Read the model definition and answer for the solid it produces. Units are mm, in the model's axes. Face numbers are marked on the shaded views. A direction names the side the tool comes from. Coordinates: 2 decimals unless noted, no trailing zeros. Loops run counter-clockwise (first coordinate to the right, second up) from the corner with the lowest first, then second, coordinate; pieces in that order, holes last. Notation, with made-up numbers: M -19,-20 L -5,-20 A26 ccw -5,-6 Z; hole C -12.5,36 d10. An arc over 180 degrees is marked long. Put each result on its own line as item: value.
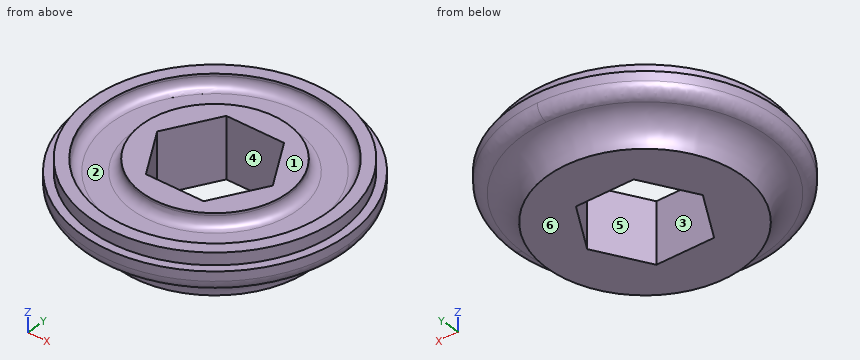
from build123d import *

# Parameters (mm, degrees)
SKETCH1_R                         = 17.4625
HEX_AXEL_CUTOUT_OUTSIDE_RIM_DEPTH = 15.875
SKETCH3_R                         = 19.05
SKETCH3_R_2                       = 16.383
PIPE_STEP_DEPTH                   = 1.5875
SKETCH5_R                         = 14.7955
SKETCH5_R_2                       = 9.525
SPOKE_STEP_DEPTH                  = 1.5875
FILLET1_R                         = 1.27
FILLET2_R                         = 1.5875
SKETCH7_W                         = 50.409195303
SKETCH7_H                         = 73.287011446
MIDCUT_DEPTH                      = 8.9375


with BuildPart() as part:
    # Sketch1 → Hex Axel Cutout & Outside Rim (new body)
    with BuildSketch(Plane.XY):
        Circle(SKETCH1_R)
        Polygon((-7.522989478, 0), (-3.761494739, -6.5151), (3.761494739, -6.5151), (7.522989478, 0), (3.761494739, 6.5151), (-3.761494739, 6.5151), align=None, mode=Mode.SUBTRACT)
    extrude(amount=HEX_AXEL_CUTOUT_OUTSIDE_RIM_DEPTH)

    # Sketch3 → Pipe Step (cut)
    with BuildSketch(Plane.XY.offset(15.875)):
        Circle(SKETCH3_R)
        Circle(SKETCH3_R_2, mode=Mode.SUBTRACT)
    pipe_step = extrude(amount=-PIPE_STEP_DEPTH, mode=Mode.SUBTRACT)

    # Step Mirror: Pipe Step across plane
    add(pipe_step.mirror(Plane.XY.offset(7.9375)), mode=Mode.SUBTRACT)

    # Sketch4 → Poly Cord Groove (revolve, cut)
    with BuildSketch(Plane(origin=(0, 0, 0), x_dir=(0, 0, -1), z_dir=(1, 0, 0))):
        with BuildLine():
            Line((-4.3815, 16.331738244), (-4.3815, 17.4625))
            Line((-4.3815, 17.4625), (-11.4935, 17.4625))
            Line((-11.4935, 17.4625), (-11.4935, 16.331738244))
            ThreePointArc((-11.4935, 16.331738244), (-7.9375, 12.775738244), (-4.3815, 16.331738244))
        make_face()
    revolve(axis=Axis((0, 0, 14.2875), (0, 0, -1)), mode=Mode.SUBTRACT)

    # Sketch5 → Spoke Step (cut)
    with BuildSketch(Plane(origin=(0, 0, 0), x_dir=(-1, 0, 0), z_dir=(0, 0, -1))):
        Circle(SKETCH5_R)
        Circle(SKETCH5_R_2, mode=Mode.SUBTRACT)
    spoke_step = extrude(amount=-SPOKE_STEP_DEPTH, mode=Mode.SUBTRACT)

    # Spoke Step Mirror: Spoke Step across plane
    add(spoke_step.mirror(Plane.XY.offset(7.9375)), mode=Mode.SUBTRACT)

    # Fillet1
    fillet1_edges = [part.edges().sort_by_distance(p)[0] for p in [
        (14.7955, 0, 1.5875),
        (9.525, 0, 1.5875),
        (14.7955, 0, 14.2875),
        (9.525, 0, 14.2875),
    ]]
    fillet(fillet1_edges, radius=FILLET1_R)

    # Fillet2
    fillet2_edges = [part.edges().sort_by_distance(p)[0] for p in [
        (-17.4625, 0, 4.3815),
        (-17.4625, 0, 11.4935),
    ]]
    fillet(fillet2_edges, radius=FILLET2_R)

    # Sketch7 → MidCut (cut, through all)
    with BuildSketch(Plane.XY.offset(7.9375)):
        with Locations((-1.207308933, -3.38321392)):
            Rectangle(SKETCH7_W, SKETCH7_H)
    extrude(amount=-MIDCUT_DEPTH, mode=Mode.SUBTRACT)


solid = part.part
1) Find section B-B, the plane z = 9.5. Write down the section's boundary in (x, y), plus the area to 3 significant figures.
Answer list:
outline: C 0,0 d26.27; hole M -7.52,0 L -3.76,-6.52 L 3.76,-6.52 L 7.52,0 L 3.76,6.52 L -3.76,6.52 Z
area: 395 mm^2
2) Given pin 1 Ø4 at (y, z) = (7.5, 9) entering from +X; pin 2 Ø2.5 at (x, z) = (2, 13) entering from -Y, each flat-ended and moving along its own axis, determine where each tip first touches the part or whether it passes through.
Answer list:
pin 1: stops at x = 12.61
pin 2: stops at y = -17.45
3) Determine the mould class of the marked faces 4, 5 and 6 for opening direction X: released by +X, released by -X, zero draft, split by the parting line, or undercut.
Answer list:
face 4: undercut
face 5: undercut
face 6: zero draft
4) Straight lines are drawn through the part: line 1 (Y direction, x = 0, z = 15.7) (1 decimal); line 2 (Y direction, x = -3.5, z = 15.25); line 3 (Z direction, x = 9, y = -9). For each, find the intervals that lie inside material, in ascending order. Write a range as [from, to].
Answer list:
line 1: y = [-16.4, -14.8], [-9.5, -6.5], [6.5, 9.5], [14.8, 16.4]
line 2: y = [-16, -14.34], [-8.9, -6.52], [6.52, 8.9], [14.34, 16]
line 3: z = [7.94, 14.29]
5) Which of the six approach directions +Z, -Z, +X, -X, +Y, -Y give full straight-line access (tool end or side, diameter ignored) to the marked faces 1, 2 and 3?
Answer list:
face 1: +Z, +X, -X, +Y, -Y
face 2: +Z
face 3: +Z, -Z
6) Find section A-A, the plane z = 15. Write down the section's boundary in (x, y), plus the area to 3 significant figures.
Answer list:
outline: C 0,0 d32.77; C 0,0 d19.31; hole C 0,0 d29.33; hole M -7.52,0 L -3.76,-6.52 L 3.76,-6.52 L 7.52,0 L 3.76,6.52 L -3.76,6.52 Z
area: 313 mm^2
